Read the model definition and answer for the solid it produces. Units are mm, in the model's axes. Face numbers are marked on the shaded views. A direction names the side the tool comes from. Coordinates: 2 decimals unless noted, no trailing zeros. Loops run counter-clockwise (first coordinate to the right, second up) from the corner with the lowest first, then second, coordinate; pieces in that order, holes last. Notation, with made-up numbers: (25, 44.25) - (83, 44.25) arc R18 cw to (83, 66.25) - close; hole circle Ø9 at (64.25, 59). An arc over 180 degrees is marked (long way). Use CSV: the item, a comma, the result in double quotes.
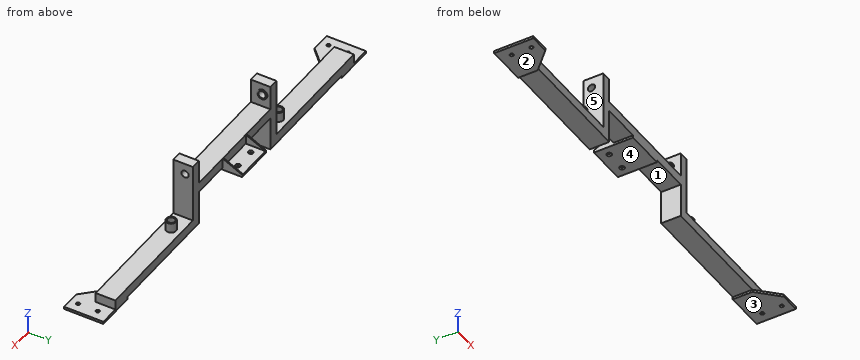
```python
from build123d import *

# Parameters (mm, degrees)
F0_W      = 355.6
F0_H      = 50.8
F1_DEPTH  = 25.4
F3_DEPTH  = 6.35
F4_R      = 4.7625
F5_DEPTH  = 25.4
F6_R      = 12.7
F6_R_2    = 9.525
F7_DEPTH  = 25.4
F8_W      = 25.4
F8_H      = 50.8
F9_DEPTH  = 152.4
F10_W     = 50.8
F10_H     = 25.4
F11_DEPTH = 152.4
F12_R     = 12.7
F12_R_2   = 9.525
F13_DEPTH = 2.54
F14_R     = 9.525
F15_DEPTH = 25.4
F16_W     = 50.8
F16_H     = 101.6
F17_DEPTH = 6.35
F18_R     = 6.35
F19_DEPTH = 25.4
F20_W     = 50.8
F20_H     = 6.35
F21_DEPTH = 3.175
F24_W     = 44.704
F24_H     = 19.304
F25_DEPTH = 327.025


with BuildPart() as f1:
    # F0 (on Top) → F1 (new body)
    with BuildSketch(Plane.XY):
        with Locations((177.8, 11.7930904027)):
            Rectangle(F0_W, F0_H)
    extrude(amount=F1_DEPTH)

    # F2 (on Top) → F3 (join)
    with BuildSketch(Plane.XY):
        Polygon((355.6, 37.1930904027), (304.8, 37.1930904027), (304.8, -13.6069095973), (355.6, -64.4069095973), (406.4, -64.4069095973), (406.4, 37.1930904027), align=None)
    extrude(amount=-F3_DEPTH)

    # F4 (on face) → F5 (cut)
    with BuildSketch(Plane.XY):
        with Locations((381, -43.7694095973)):
            Circle(F4_R)
        with Locations((381, 7.0305904027)):
            Circle(F4_R)
    extrude(amount=-F5_DEPTH, mode=Mode.SUBTRACT)

    # F6 (on face) → F7 (join)
    with BuildSketch(Plane.XY.offset(25.4)):
        with Locations((76.2, 11.7930904027)):
            Circle(F6_R)
        with Locations((76.2, 11.7930904027)):
            Circle(F6_R_2, mode=Mode.SUBTRACT)
    extrude(amount=F7_DEPTH)

    # F8 (on face) → F9 (join)
    with BuildSketch(Plane.XY.offset(25.4)):
        with Locations((12.7, 11.7930904027)):
            Rectangle(F8_W, F8_H)
    extrude(amount=F9_DEPTH)

    # F10 (on face) → F11 (join)
    with BuildSketch(Plane(origin=(0, 0, 0), x_dir=(0, -1, 0), z_dir=(-1, 0, 0))):
        with Locations((-11.7930904027, 101.6)):
            Rectangle(F10_W, F10_H)
    extrude(amount=F11_DEPTH)

    # F12 (on face) → F13 (join)
    with BuildSketch(Plane(origin=(0, 0, 0), x_dir=(0, -1, 0), z_dir=(-1, 0, 0))):
        with Locations((-16.9099774212, 149.1121947765)):
            Circle(F12_R)
        with Locations((-16.9099774212, 149.1121947765)):
            Circle(F12_R_2, mode=Mode.SUBTRACT)
    extrude(amount=F13_DEPTH)

    # F14 (on face) → F15 (cut)
    with BuildSketch(Plane(origin=(0, 0, 0), x_dir=(0, -1, 0), z_dir=(-1, 0, 0))):
        with Locations((-16.9099774212, 149.1121947765)):
            Circle(F14_R)
    extrude(amount=-F15_DEPTH, mode=Mode.SUBTRACT)

    # F16 (on face) → F17 (join)
    with BuildSketch(Plane(origin=(0, 0, 88.9), x_dir=(1, 0, 0), z_dir=(0, 0, -1))):
        with Locations((-127, -37.1930904027)):
            Rectangle(F16_W, F16_H)
    extrude(amount=F17_DEPTH)

    # F18 (on face) → F19 (cut)
    with BuildSketch(Plane.XY.offset(88.9)):
        with Locations((-124.9504238367, 62.5930904027)):
            Circle(F18_R)
    extrude(amount=-F19_DEPTH, mode=Mode.SUBTRACT)

    # F20 (on face) → F21 (join)
    with BuildSketch(Plane.YZ.offset(-101.6)):
        Polygon((37.1930904027, 88.9), (87.9930904027, 88.9), (37.1930904027, 114.3), align=None)
        with Locations((62.5930904027, 85.725)):
            Rectangle(F20_W, F20_H)
    extrude(amount=-F21_DEPTH)

    # F22: F1 across face


with BuildPart() as f1_1:
    add(f1.part)
    add(f1.part.mirror(Plane(origin=(-152.4, 20.2597570693, 96.3083333333), x_dir=(0, -1, 0), z_dir=(-1, 0, 0))))

    # F24 (on offset) → F25 (cut, through all)
    with BuildSketch(Plane.YZ.offset(352.425)):
        with Locations((11.7930904027, 12.7)):
            Rectangle(F24_W, F24_H)
    extrude(amount=-F25_DEPTH, mode=Mode.SUBTRACT)


solid = f1_1.part
```
Q1. Given P1, Ø16, axis at y = 45, z = 92, coming from the -X side; P2, Ø7.5, axis at x = 381, y = -43.77, coming from the -Z side; P3, Ø25, axis at y = 16.91, z = 149.11, coming from the +X side; P4, Ø7.5, axis at y = 51.5, z = 98.5, coming from the +X side, each flat-ended and moving along its own axis, determine where each tip first touches the part or whether it passes through.
Reported:
P1,"stops at x = -330.2"
P2,"passes through"
P3,"stops at x = 25.4"
P4,"stops at x = -101.6"
Q2. A tool of negligible diameter and unlimited length cuts with its end or side. For the marked faces 3, 4 and 5, from which of +Z, -Z, +X, -X, +Y, -Y can it reach the whole face along a straight path? Write none if from no direction.
Reported:
face 3,"-Z, +X, -X, +Y, -Y"
face 4,"-Z, +Y, -Y"
face 5,"+Z, +Y, -Y"
Q3. The part is cut by section C-C on x = 76.2. Determine the outline of the cut face in (y, z), and give its area (3 significant figures).
Reported:
outline,"(-13.61, 0) - (37.19, 0) - (37.19, 25.4) - (24.49, 25.4) - (24.49, 50.8) - (21.32, 50.8) - (21.32, 25.4) - (2.27, 25.4) - (2.27, 50.8) - (-0.91, 50.8) - (-0.91, 25.4) - (-13.61, 25.4) - close; hole (-10.56, 3.05) - (34.15, 3.05) - (34.15, 22.35) - (-10.56, 22.35) - close"
area,"589 mm²"
Q4. The part is cut by section B-B on x = -381. Determine the outline of the cut face in (y, z).
Reported:
outline,"(-13.61, 0) - (37.19, 0) - (37.19, 25.4) - (24.49, 25.4) - (24.49, 50.8) - (21.32, 50.8) - (21.32, 25.4) - (2.27, 25.4) - (2.27, 50.8) - (-0.91, 50.8) - (-0.91, 25.4) - (-13.61, 25.4) - close"
Q5. The part is cut by section A-A on x = 195. Determine the outline of the cut face in (y, z), and give its area (3 significant figures).
Reported:
outline,"(-13.61, 0) - (37.19, 0) - (37.19, 25.4) - (-13.61, 25.4) - close; hole (-10.56, 3.05) - (34.15, 3.05) - (34.15, 22.35) - (-10.56, 22.35) - close"
area,"427 mm²"
Q6. For a pull along X with two mould halves and no side action, classify the marked faces 1 and 2 as +X half, -X half, draft (parallel to the pull), parting line (faces both ways), or undercut.
Reported:
face 1,"undercut"
face 2,"draft"
Q7. Find the intervals of material crossed by probe 1 along Y at (x, z) = (-685, -4); probe 2 along Y at (x, z) = (381, -3); probe 3 along X at (y, z) = (3, 13) (3 decimals), in increasing order. Write a range as [from, to].
Reported:
probe 1,"y = [-64.41, -48.46], [-39.07, 2.34], [11.73, 37.19]"
probe 2,"y = [-64.41, -48.53], [-39.01, 2.27], [11.79, 37.19]"
probe 3,"x = [-660.4, -304.8], [0, 25.4], [352.425, 355.6]"
